CAD build for the part. Positions are in the model's coordinates, mm. Give positions to 0.01 mm unless a question says otherwise; leave off trailing zeros. Write each loop counter-clockwise with the first axis right and the second up, starting at its lowest first coordinate (ties: lowest second). Pieces come first, ordered by that corner, then holes. Notation, with made-up numbers: (65, 77) -> (77, 77) arc R22 cw to (77, 115) -> close; hole circle Ø11 at (-38, -14.75). An arc over 180 degrees is marked (long way). Answer as a JSON object with one key per item and string values.
```python
from build123d import *

# Parameters (mm, degrees)
SKETCH_1_R          = 25
SKETCH_1_R_2        = 2.1
SKETCH_1_W          = 4
SKETCH_1_H          = 1.5
EXTRUDE_1_DEPTH     = 4
SKETCH_3_R          = 1.5
SKETCH_3_R_2        = 2
SKETCH_3_W          = 8.03
SKETCH_3_H          = 4.03
SKETCH_3_W_2        = 4.03
SKETCH_3_H_2        = 8.03
CUT_EXTRUDE_2_DEPTH = 4
SKETCH_7_R          = 3
CUT_EXTRUDE_3_DEPTH = 10


with BuildPart() as part:
    # 草图1 → 凸台-拉伸1 (new body)
    with BuildSketch(Plane.XY):
        Polygon((151.457142857, -41.187142857), (151.457142857, 108.812857143), (-148.542857143, 108.812857143), (-148.542857143, -191.187142857), (151.457142857, -191.187142857), align=None)
        with Locations((1.457142857, -41.187142857)):
            Circle(SKETCH_1_R, mode=Mode.SUBTRACT)
        with Locations((25.027142857, -17.617142857)):
            Circle(SKETCH_1_R_2, mode=Mode.SUBTRACT)
        with Locations((25.027142857, -64.757142857)):
            Circle(SKETCH_1_R_2, mode=Mode.SUBTRACT)
        with Locations((-22.112857143, -64.757142857)):
            Circle(SKETCH_1_R_2, mode=Mode.SUBTRACT)
        with Locations((-22.112857143, -17.617142857)):
            Circle(SKETCH_1_R_2, mode=Mode.SUBTRACT)
        with Locations((65.457142857, 98.062857143)):
            Rectangle(SKETCH_1_W, SKETCH_1_H, mode=Mode.SUBTRACT)
        with Locations((-62.542857143, 98.062857143)):
            Rectangle(SKETCH_1_W, SKETCH_1_H, mode=Mode.SUBTRACT)
    extrude(amount=EXTRUDE_1_DEPTH)

    # 草图3 → 切除-拉伸2 (cut)
    with BuildSketch(Plane.XY.offset(4)):
        with Locations((1.457142857, -185.187142857)):
            Circle(SKETCH_3_R)
        with Locations((67.457142857, -185.187142857)):
            Circle(SKETCH_3_R)
        with Locations(Location((-64.542857143, -185.187142857, 0), (0, 0, 180))):
            Circle(SKETCH_3_R)
        with Locations(Location((-142.542857143, 24.812857143, 0), (0, 0, 180))):
            Circle(SKETCH_3_R)
        with Locations((-142.542857143, -41.187142857)):
            Circle(SKETCH_3_R)
        with Locations((-142.542857143, -107.187142857)):
            Circle(SKETCH_3_R)
        with Locations(Location((67.457142857, 102.812857143, 0), (0, 0, 180))):
            Circle(SKETCH_3_R)
        with Locations((1.457142857, 102.812857143)):
            Circle(SKETCH_3_R)
        with Locations((-64.542857143, 102.812857143)):
            Circle(SKETCH_3_R)
        with Locations(Location((145.457142857, -107.187142857, 0), (0, 0, 180))):
            Circle(SKETCH_3_R)
        with Locations((145.457142857, -41.187142857)):
            Circle(SKETCH_3_R)
        with Locations((145.457142857, 24.812857143)):
            Circle(SKETCH_3_R)
        with Locations((50.957142857, -170.187142857)):
            Circle(SKETCH_3_R_2)
        with Locations(Location((-48.042857143, -170.187142857, 0), (0, 0, 180))):
            Circle(SKETCH_3_R_2)
        with Locations((-31.542857143, -155.187142857)):
            Circle(SKETCH_3_R_2)
        with Locations(Location((34.457142857, -155.187142857, 0), (0, 0, 180))):
            Circle(SKETCH_3_R_2)
        with Locations((1.457142857, -88.187142857)):
            Circle(SKETCH_3_R_2)
        with Locations((-31.776875859, -74.421161573)):
            Circle(SKETCH_3_R_2)
        with Locations((-45.542857143, -41.187142857)):
            Circle(SKETCH_3_R_2)
        with Locations((-31.776875859, -7.953124141)):
            Circle(SKETCH_3_R_2)
        with Locations((1.457142857, 5.812857143)):
            Circle(SKETCH_3_R_2)
        with Locations((34.691161573, -7.953124141)):
            Circle(SKETCH_3_R_2)
        with Locations((48.457142857, -41.187142857)):
            Circle(SKETCH_3_R_2)
        with Locations((34.691161573, -74.421161573)):
            Circle(SKETCH_3_R_2)
        with Locations((1.457142857, -125.187142857)):
            Circle(SKETCH_3_R_2)
        with Locations((100.457142857, -185.187142857)):
            Rectangle(SKETCH_3_W, SKETCH_3_H)
        with Locations((34.457142857, -185.187142857)):
            Rectangle(SKETCH_3_W, SKETCH_3_H)
        with Locations((-31.542857143, -185.187142857)):
            Rectangle(SKETCH_3_W, SKETCH_3_H)
        with Locations((-97.542857143, -185.187142857)):
            Rectangle(SKETCH_3_W, SKETCH_3_H)
        with Locations((-142.542857143, 57.812857143)):
            Rectangle(SKETCH_3_W_2, SKETCH_3_H_2)
        with Locations((-142.542857143, -8.187142857)):
            Rectangle(SKETCH_3_W_2, SKETCH_3_H_2)
        with Locations((-142.542857143, -74.187142857)):
            Rectangle(SKETCH_3_W_2, SKETCH_3_H_2)
        with Locations((-142.542857143, -140.187142857)):
            Rectangle(SKETCH_3_W_2, SKETCH_3_H_2)
        with Locations((100.457142857, 102.812857143)):
            Rectangle(SKETCH_3_W, SKETCH_3_H)
        with Locations((34.457142857, 102.812857143)):
            Rectangle(SKETCH_3_W, SKETCH_3_H)
        with Locations((-31.542857143, 102.812857143)):
            Rectangle(SKETCH_3_W, SKETCH_3_H)
        with Locations((-97.542857143, 102.812857143)):
            Rectangle(SKETCH_3_W, SKETCH_3_H)
        with Locations((145.457142857, -140.187142857)):
            Rectangle(SKETCH_3_W_2, SKETCH_3_H_2)
        with Locations((145.457142857, -74.187142857)):
            Rectangle(SKETCH_3_W_2, SKETCH_3_H_2)
        with Locations((145.457142857, -8.187142857)):
            Rectangle(SKETCH_3_W_2, SKETCH_3_H_2)
        with Locations((145.457142857, 57.812857143)):
            Rectangle(SKETCH_3_W_2, SKETCH_3_H_2)
    extrude(amount=-CUT_EXTRUDE_2_DEPTH, mode=Mode.SUBTRACT)

    # 草图7 → 切除-拉伸3 (cut)
    with BuildSketch(Plane.XY.offset(4)):
        with Locations((-88.542857143, -171.187142857)):
            Circle(SKETCH_7_R)
        with Locations((91.457142857, -171.187142857)):
            Circle(SKETCH_7_R)
        with Locations((-128.542857143, 48.812857143)):
            Circle(SKETCH_7_R)
        with Locations((-128.542857143, -131.187142857)):
            Circle(SKETCH_7_R)
        with Locations((91.457142857, 88.812857143)):
            Circle(SKETCH_7_R)
        with Locations((-88.542857143, 88.812857143)):
            Circle(SKETCH_7_R)
        with Locations((131.457142857, -131.187142857)):
            Circle(SKETCH_7_R)
        with Locations((131.457142857, 48.812857143)):
            Circle(SKETCH_7_R)
    extrude(amount=-CUT_EXTRUDE_3_DEPTH, mode=Mode.SUBTRACT)


solid = part.part
```
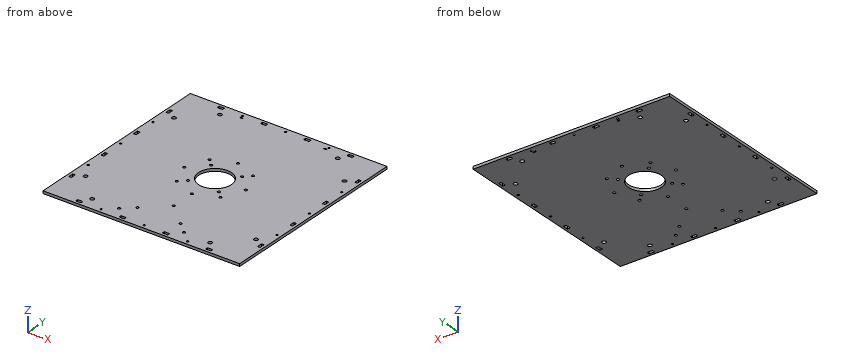
1) Slice it at A-A (y = -31.5). List the corners of the cut face in (x, z).
Model answer:
{"outline": "(-148.54, 0) -> (-21.59, 0) -> (-21.59, 4) -> (-148.54, 4) -> close; (24.5, 0) -> (151.46, 0) -> (151.46, 4) -> (24.5, 4) -> close"}
2) Pin check, flat tip, straight feed: pin 1 (4 mm diameter, centred on x = 46.5, y = -38, fed in from -Z). Stop position of the tip, or through.
Model answer:
{"pin 1": "stops at z = 0"}
3) Slice it at C-C (z = 2.25). State how many separate pieces and enclosed holes the cut face has, then the cut area to 3 significant figures.
Model answer:
{"separate pieces": "1", "enclosed holes": "56", "area": "87,000 mm2"}
4) Wall check: probe 1 along Y at (x, z) = (30.5, 2.05); probe 2 along X at (y, z) = (-8.5, 1.7); probe 3 along Y at (x, z) = (89, 2.15). Give the ranges that are in metal, low to high.
Model answer:
{"probe 1": "y = -191.19 to -187.2, -183.17 to 100.8, 104.83 to 108.81", "probe 2": "x = -148.54 to -144.56, -140.53 to -33.7, -29.85 to 32.77, 36.61 to 143.44, 147.47 to 151.46", "probe 3": "y = -191.19 to -172.91, -169.47 to 87.09, 90.53 to 108.81"}
5) Slice it at B-B (x = -15). List the corners of the cut face in (y, z), then the cut area to 3 significant figures.
Model answer:
{"outline": "(-191.19, 0) -> (-60.01, 0) -> (-60.01, 4) -> (-191.19, 4) -> close; (-22.37, 0) -> (108.81, 0) -> (108.81, 4) -> (-22.37, 4) -> close", "area": "1,050 mm2"}
